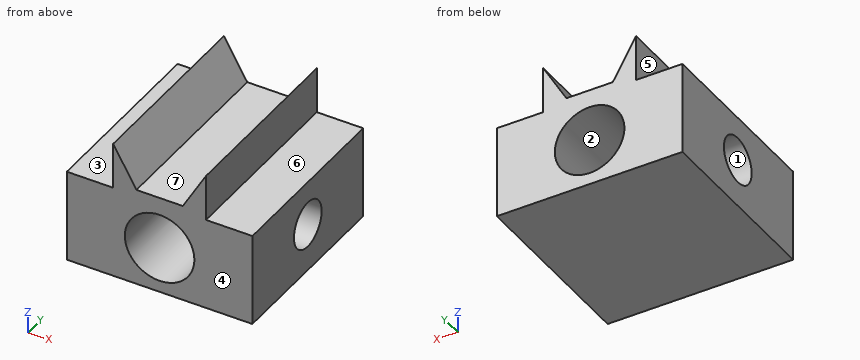
from build123d import *

# Parameters (mm, degrees)
F0_W     = 101.6
F0_H     = 50.8
F1_DEPTH = 101.6
F2_W     = 50.8
F2_H     = 101.6
F3_DEPTH = 25.4
F5_DEPTH = 101.6
F6_R     = 19.05
F7_DEPTH = 101.6
F8_R     = 12.7
F9_DEPTH = 101.6


with BuildPart() as f1:
    # F0 (on Front) → F1 (new body)
    with BuildSketch(Plane.XZ):
        with Locations((50.8, 25.4)):
            Rectangle(F0_W, F0_H)
    extrude(amount=F1_DEPTH)

    # F2 (on face) → F3 (join)
    with BuildSketch(Plane.XY.offset(50.8)):
        with Locations((50.8, -50.8)):
            Rectangle(F2_W, F2_H)
    extrude(amount=F3_DEPTH)

    # F4 (on face) → F5 (cut)
    with BuildSketch(Plane.XZ.offset(101.6)):
        Polygon((76.2, 76.2), (25.4, 76.2), (38.1, 54.202955), (63.5, 54.202955), align=None)
    extrude(amount=-F5_DEPTH, mode=Mode.SUBTRACT)

    # F6 (on face) → F7 (cut)
    with BuildSketch(Plane.XZ.offset(101.6)):
        with Locations((50.8, 25.4)):
            Circle(F6_R)
    extrude(amount=-F7_DEPTH, mode=Mode.SUBTRACT)

    # F8 (on face) → F9 (cut)
    with BuildSketch(Plane(origin=(0, 0, 0), x_dir=(0, -1, 0), z_dir=(-1, 0, 0))):
        with Locations((50.8, 26.370544)):
            Circle(F8_R)
    extrude(amount=-F9_DEPTH, mode=Mode.SUBTRACT)


solid = f1.part
Verification items for the finished model (mm, model axes). Face numbers are marked on the shaded views. A direction names the side the tool comes from. Give positions to 0.01 mm unless a question says otherwise; leave off trailing zeros. Loops run counter-clockwise (first coordinate to the right, second up) from the corner with the lowest first, then second, coordinate; pieces in that order, holes last.
1. Cross-section at A-A on x = 50.8. Record the cut outline in (y, z).
Derived:
outline: (-101.6, 0) - (0, 0) - (0, 6.35) - (-101.6, 6.35) - close; (-101.6, 44.45) - (0, 44.45) - (0, 54.2) - (-101.6, 54.2) - close
2. Material ranges on probe 1 along Z at (x, y) = (24, -50.8); probe 2 along Z at (x, y) = (23, -50); probe 3 along X at (y, z) = (-59, 12.5), recorded low to high.
Derived:
probe 1: z = 0 to 13.67, 39.07 to 50.8
probe 2: z = 0 to 13.7, 39.05 to 50.8
probe 3: x = 0 to 36.78, 64.82 to 101.6
3. Tool access check on the marked faces 5, 6 and 7. Record the directions out of +Z, -Z, +X, -X, +Y, -Y that give a thin tool (end or side, any length) a straight path to the whole face; none if there is none.
Derived:
face 5: +Z, -X, +Y, -Y
face 6: +Z, +X, +Y, -Y
face 7: +Z, +Y, -Y
4. Go/stop test with flat-tipped pins: P1, Ø7.5, axis at x = 8, y = -48, coming from the +Z side; P2, Ø12.5, axis at y = -36.5, z = 60, coming from the +X side; P3, Ø20.5, axis at y = -50.8, z = 26.37, coming from the -X side; P4, Ø12.5, axis at x = 56.5, y = -67.5, coming from the +Z side. Record where each tip stops, or that it passes through.
Derived:
P1: stops at z = 50.8
P2: stops at x = 76.2
P3: passes through
P4: stops at z = 54.2
5. Cross-section at B-B on z = 20.5. Record the cut outline in (x, y), and give its area (3 significant figures).
Derived:
outline: (0, -101.6) - (32.39, -101.6) - (32.39, -62.06) - (0, -62.06) - close; (0, -39.54) - (32.39, -39.54) - (32.39, 0) - (0, 0) - close; (69.21, -101.6) - (101.6, -101.6) - (101.6, -62.06) - (69.21, -62.06) - close; (69.21, -39.54) - (101.6, -39.54) - (101.6, 0) - (69.21, 0) - close
area: 5,120 mm2
6. Release check for a two-part mould opening along Z. For the marked faces 1, 2, 3 and 4 record: +Z half, -Z half, draft (parallel to the pull), parting line (faces both ways), or undercut.
Derived:
face 1: undercut
face 2: undercut
face 3: +Z half
face 4: draft
7. Cross-section at D-D on z = 56.5. Record the cut outline in (x, y), and give its area (3 significant figures).
Derived:
outline: (25.4, -101.6) - (36.77, -101.6) - (36.77, 0) - (25.4, 0) - close; (64.83, -101.6) - (76.2, -101.6) - (76.2, 0) - (64.83, 0) - close
area: 2,310 mm2
8. Cross-section at C-C on y = -9. Record the cut outline in (x, z), and give its area (3 significant figures).
Derived:
outline: (0, 0) - (101.6, 0) - (101.6, 50.8) - (76.2, 50.8) - (76.2, 76.2) - (63.5, 54.2) - (38.1, 54.2) - (25.4, 76.2) - (25.4, 50.8) - (0, 50.8) - close; hole circle Ø38.1 at (50.8, 25.4)
area: 4,470 mm2
